```python
from build123d import *

# Parameters (mm, degrees)
CROQUIS1_W              = 70
CROQUIS1_H              = 70
SALIENTE_EXTRUIR1_DEPTH = 6
SALIENTE_EXTRUIR2_DEPTH = 52
CROQUIS4_R              = 2.25
CORTAR_EXTRUIR1_DEPTH   = 83.498484835
CHAFL_N1_SIZE           = 2.25


with BuildPart() as part:
    # Croquis1 → Saliente-Extruir1 (new body)
    with BuildSketch(Plane(origin=(0, 0, 0), x_dir=(1, 0, 0), z_dir=(0, 1, 0))):
        Rectangle(CROQUIS1_W, CROQUIS1_H)
    extrude(amount=SALIENTE_EXTRUIR1_DEPTH)

    # Croquis2 → Revolución1 (revolve)
    with BuildSketch(Plane.XY, mode=Mode.PRIVATE) as revoluci_n1_sk:
        Polygon((7.3, 6), (12, 6), (12, 66), (11, 66), (7.3, 58), align=None)
    revolve(revoluci_n1_sk.sketch.rotate(Axis((0, 0, 0), (0, 1, 0)), 90), axis=Axis((0, 0, 0), (0, 1, 0)))

    # Croquis3 → Saliente-Extruir2 (add)
    with BuildSketch(Plane(origin=(0, 6, 0), x_dir=(1, 0, 0), z_dir=(0, 1, 0))):
        with BuildLine():
            Line((6.3, -3.687817783), (6.3, 3.687817783))
            ThreePointArc((6.3, 3.687817783), (7.3, 0), (6.3, -3.687817783))
        make_face()
    extrude(amount=SALIENTE_EXTRUIR2_DEPTH)

    # Croquis4 → Cortar-Extruir1 (cut, through all)
    with BuildSketch(Plane(origin=(0, 0, 0), x_dir=(1, 0, 0), z_dir=(0, 1, 0))):
        with Locations(Location((27, 27, 0), (0, 0, 270))):
            Circle(CROQUIS4_R)
        with Locations(Location((27, -27, 0), (0, 0, 270))):
            Circle(CROQUIS4_R)
        with Locations(Location((-27, 27, 0), (0, 0, 270))):
            Circle(CROQUIS4_R)
        with Locations(Location((-27, -27, 0), (0, 0, 270))):
            Circle(CROQUIS4_R)
    extrude(amount=CORTAR_EXTRUIR1_DEPTH, mode=Mode.SUBTRACT)

    # Chaflán1
    chafl_n1_edges = [part.edges().sort_by_distance(p)[0] for p in [
        (27, 6, 24.75),
        (-27, 6, -29.25),
        (-27, 6, 24.75),
        (27, 6, -29.25),
    ]]
    chamfer(chafl_n1_edges, length=CHAFL_N1_SIZE)


solid = part.part
```
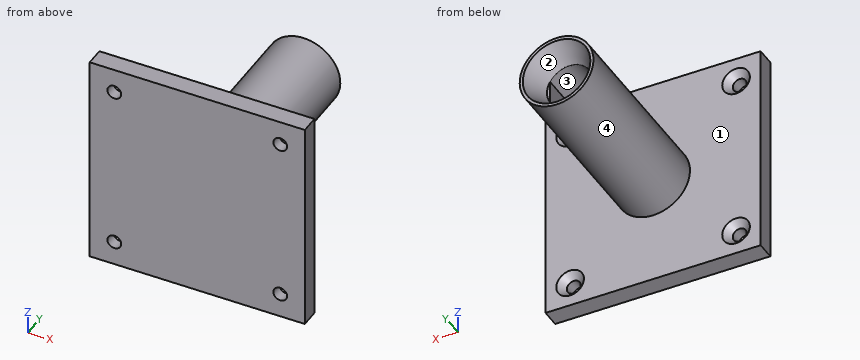
Could you check a few things on this model? Use its own coordinates, in mm. Face numbers are marked on the shaded views. Coordinates: 2 decimals unless noted, no trailing zeros. Order: outer loops, then holes, each group sorted by start corner. A loop starts at its lowest first (then second) coordinate and runs counter-clockwise, first axis right, second up. Notation, with made-up numbers: M 25,17 L 60,17 A13 ccw 60,41 Z; hole C 30.5,-29.75 d6. An arc over 180 degrees is marked long. Use a Markdown table: item, result. Add a question column.
Q1. We'd pull the mould along Z, two halves only. Please class the marked faces 1, 2, 3 and 4: pulls with the +Z half, pulls with the -Z half, needs draft (parallel to the pull), parting line crosses it, or undercut.
Q2. I want a section at A-A on x = -27. List the corners of the cut face in (y, z) for me.
Q3. I want a section at B-B on z = 27. List the corners of the cut face in (x, y) for me.
Q4. If I drill on L1, parallel to X at y = 1, z = -27; L2, parallel to Y at x = -32, z = 18.5, over which ranges is the centre line in solid material (lowest first)?
Q5. I want a section at C-C on z = 0. List the corners of the cut face in (x, y) for me.
Q6. I want a section at D-D on y = 55. List the corners of the cut face in (x, z) for me, then the cut area to 3 significant figures.
Q7. I'm going to push flat-ended pins straight in: pin 1 (12 mm diameter, centred on y = 51, z = -4.5, fed in from +X); pin 2 (4 mm diameter, centred on x = -1, z = -1, fed in from +Y); pin 3 (2 mm diameter, centred on y = 23.5, z = 1.5, fed in from -X). Where does each tip first touch, or does it pass through?
Checked values:
| question | item | result |
|---|---|---|
| 1 | face 1 | needs draft |
| 1 | face 2 | undercut |
| 1 | face 3 | undercut |
| 1 | face 4 | parting line crosses it |
| 2 | outline | M 0,-35 L 6,-35 L 6,-31.5 L 3.75,-29.25 L 0,-29.25 Z; M 0,-24.75 L 3.75,-24.75 L 6,-22.5 L 6,22.5 L 3.75,24.75 L 0,24.75 Z; M 0,29.25 L 3.75,29.25 L 6,31.5 L 6,35 L 0,35 Z |
| 3 | outline | M -35,0 L -29.25,0 L -29.25,3.75 L -31.5,6 L -35,6 Z; M -24.75,0 L 24.75,0 L 24.75,3.75 L 22.5,6 L -22.5,6 L -24.75,3.75 Z; M 29.25,0 L 35,0 L 35,6 L 31.5,6 L 29.25,3.75 Z |
| 4 | L1 | -35 to -29.25, -24.75 to 24.75, 29.25 to 35 |
| 4 | L2 | 0 to 6 |
| 5 | outline | M -35,0 L 35,0 L 35,6 L 12,6 L 12,66 L 11,66 L 7.3,58 L 6.3,58 L 6.3,6 L -7.3,6 L -7.3,58 L -11,66 L -12,66 L -12,6 L -35,6 Z |
| 6 | outline | C 0,0 d24; hole M 6.3,-3.69 L 6.3,3.69 A7.3 ccw long Z |
| 6 | area | 290 mm² |
| 7 | pin 1 | x = 12 |
| 7 | pin 2 | y = 6 |
| 7 | pin 3 | x = -11.99 |
